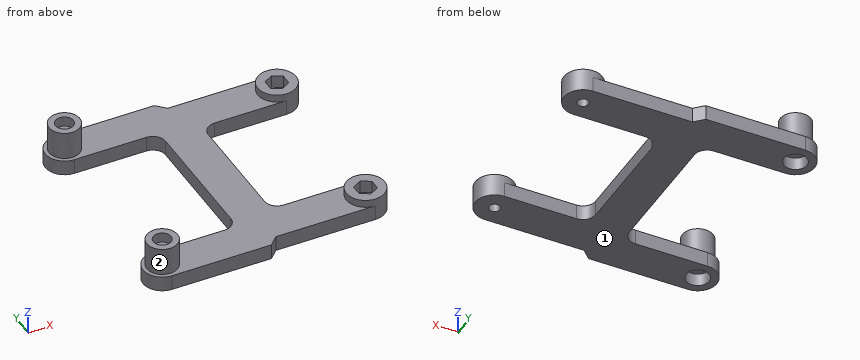
```python
from build123d import *

# Parameters (mm, degrees)
SKETCH1_R           = 4.5
SKETCH1_R_2         = 2.15
BOSS_EXTRUDE1_DEPTH = 6
BOSS_EXTRUDE2_START = -1
SKETCH2_R           = 6
SKETCH2_R_2         = 3.5
BOSS_EXTRUDE2_DEPTH = 12
BOSS_EXTRUDE3_START = -5
SKETCH3_R           = 3.5
SKETCH3_R_2         = 1.65
BOSS_EXTRUDE3_DEPTH = 8
SKETCH4_R           = 7.5
SKETCH4_R_2         = 2.15
BOSS_EXTRUDE4_DEPTH = 3
CUT_EXTRUDE1_DEPTH  = 5


with BuildPart() as part:
    # Sketch1 → Boss-Extrude1 (new body)
    with BuildSketch(Plane.XY):
        with BuildLine():
            Line((0, 82.5), (39, 82.5))
            Line((39, 82.5), (42.5, 79))
            Line((42.5, 79), (81.5, 79))
            ThreePointArc((81.5, 79), (89, 71.5), (81.5, 64))
            Line((81.5, 64), (53.25, 64))
            ThreePointArc((53.25, 64), (49.714466094, 62.535533906), (48.25, 59))
            Line((48.25, 59), (48.25, 16))
            ThreePointArc((48.25, 16), (49.714466094, 12.464466094), (53.25, 11))
            Line((53.25, 11), (81.5, 11))
            ThreePointArc((81.5, 11), (89, 3.5), (81.5, -4))
            Line((81.5, -4), (42.5, -4))
            Line((42.5, -4), (39, -7.5))
            Line((39, -7.5), (0, -7.5))
            ThreePointArc((0, -7.5), (-7.5, 0), (0, 7.5))
            Line((0, 7.5), (28.25, 7.5))
            ThreePointArc((28.25, 7.5), (31.785533906, 8.964466094), (33.25, 12.5))
            Line((33.25, 12.5), (33.25, 62.5))
            ThreePointArc((33.25, 62.5), (31.785533906, 66.035533906), (28.25, 67.5))
            Line((28.25, 67.5), (0, 67.5))
            ThreePointArc((0, 67.5), (-7.5, 75), (0, 82.5))
        make_face()
        Circle(SKETCH1_R, mode=Mode.SUBTRACT)
        with Locations(Location((0, 75, 0), (0, 0, 180))):
            Circle(SKETCH1_R, mode=Mode.SUBTRACT)
        with Locations((81.5, 71.5)):
            Circle(SKETCH1_R_2, mode=Mode.SUBTRACT)
        with Locations((81.5, 3.5)):
            Circle(SKETCH1_R_2, mode=Mode.SUBTRACT)
    extrude(amount=BOSS_EXTRUDE1_DEPTH)

    # Sketch2 → Boss-Extrude2 (add)
    # profile 1 of 2: a face of its own
    with BuildSketch(Plane.XY.offset(6).offset(BOSS_EXTRUDE2_START)):
        with Locations(Location((0, 75, 0), (0, 0, 180))):
            Circle(SKETCH2_R)
        with Locations((0, 75)):
            Circle(SKETCH2_R_2, mode=Mode.SUBTRACT)
    # profile 2 of 2: a face of its own
    with BuildSketch(Plane.XY.offset(6).offset(BOSS_EXTRUDE2_START)):
        with Locations(Location((0, 0, 0), (0, 0, 180))):
            Circle(SKETCH2_R)
        Circle(SKETCH2_R_2, mode=Mode.SUBTRACT)
    extrude(amount=BOSS_EXTRUDE2_DEPTH)

    # Sketch3 → Boss-Extrude3 (add)
    # profile 1 of 2: a face of its own
    with BuildSketch(Plane(origin=(0, 0, 0), x_dir=(-1, 0, 0), z_dir=(0, 0, -1)).offset(BOSS_EXTRUDE3_START)):
        with Locations(Location((0, 75, 0), (0, 0, 180))):
            Circle(SKETCH3_R)
        with Locations((0, 75)):
            Circle(SKETCH3_R_2, mode=Mode.SUBTRACT)
    # profile 2 of 2: a face of its own
    with BuildSketch(Plane(origin=(0, 0, 0), x_dir=(-1, 0, 0), z_dir=(0, 0, -1)).offset(BOSS_EXTRUDE3_START)):
        with Locations(Location((0, 0, 0), (0, 0, 180))):
            Circle(SKETCH3_R)
        Circle(SKETCH3_R_2, mode=Mode.SUBTRACT)
    extrude(amount=-BOSS_EXTRUDE3_DEPTH)

    # Sketch4 → Boss-Extrude4 (add)
    # profile 1 of 2: a face of its own
    with BuildSketch(Plane.XY.offset(6)):
        with Locations(Location((81.5, 3.5, 0), (0, 0, 90))):
            Circle(SKETCH4_R)
        with Locations((81.5, 3.5)):
            Circle(SKETCH4_R_2, mode=Mode.SUBTRACT)
    # profile 2 of 2: a face of its own
    with BuildSketch(Plane.XY.offset(6)):
        with Locations(Location((81.5, 71.5, 0), (0, 0, 90))):
            Circle(SKETCH4_R)
        with Locations((81.5, 71.5)):
            Circle(SKETCH4_R_2, mode=Mode.SUBTRACT)
    extrude(amount=BOSS_EXTRUDE4_DEPTH)

    # Sketch5 → Cut-Extrude1 (cut)
    with BuildSketch(Plane.XY.offset(9)):
        Polygon((77.9, 5.578460969), (81.5, 7.656921938), (85.1, 5.578460969), (85.1, 1.421539031), (81.5, -0.656921938), (77.9, 1.421539031), align=None)
        Polygon((77.9, 73.578460969), (81.5, 75.656921938), (85.1, 73.578460969), (85.1, 69.421539031), (81.5, 67.343078062), (77.9, 69.421539031), align=None)
    extrude(amount=-CUT_EXTRUDE1_DEPTH, mode=Mode.SUBTRACT)


solid = part.part
```
Geometry check sheet. Reference: the model listing, model coordinates, mm. Face numbers are marked on the shaded views. Coordinates: 2 decimals unless noted, no trailing zeros. Order: outer loops, then holes, each group sorted by start corner. A loop starts at its lowest first (then second) coordinate and runs counter-clockwise, first axis right, second up.
Q1. Draft check along Y on the marked faces 1 and 2. Enter one of: released by +Y, released by -Y, zero draft, split by the parting line, or undercut.
Reply:
face 1: zero draft
face 2: undercut
Q2. Sectioned sample at C-C on y = 25. Record the cut outline in (x, z), and give its area (3 significant figures).
Reply:
outline: (33.25, 0) - (48.25, 0) - (48.25, 6) - (33.25, 6) - close
area: 90.0 mm2
Q3. Sectioned sample at A-A on x = 60. Record the cut outline in (y, z), and give its area (3 significant figures).
Reply:
outline: (-4, 0) - (11, 0) - (11, 6) - (-4, 6) - close; (64, 0) - (79, 0) - (79, 6) - (64, 6) - close
area: 180 mm2
Q4. Depth check by flat-ended pin: pin 1 Ø8 at (x, z) = (76.5, 5.5) entering from +Y; pin 2 Ø1.8 at (x, z) = (55.5, 2.5) entering from -Y; pin 3 Ø1.5 at (x, y) = (49.5, 32) entering from -Z; pin 4 Ø2 at (x, y) = (0, -1) entering from +Z. Enter the tip coordinate at first touch or a pass-through.
Reply:
pin 1: stops at y = 79
pin 2: stops at y = -4
pin 3: passes through
pin 4: stops at z = 13
Q5. Thickness scan on probe 1 along Y at (x, z) = (0, 1.2); probe 2 along Y at (x, z) = (81.5, 2.75); probe 3 along Y at (x, z) = (74.5, 3.5). Record the ranges inside material, lowest first.
Reply:
probe 1: y = -7.5 to -4.5, 4.5 to 7.5, 67.5 to 70.5, 79.5 to 82.5
probe 2: y = -4 to 1.35, 5.65 to 11, 64 to 69.35, 73.65 to 79
probe 3: y = -4 to 11, 64 to 79
Q6. Sectioned sample at B-B on z = 1.5. Record the cut outline in (x, y).
Reply:
outline: (0, -7.5) - (39, -7.5) - (42.5, -4) - (81.5, -4) arc R7.5 ccw to (81.5, 11) - (53.25, 11) arc R5 cw to (48.25, 16) - (48.25, 59) arc R5 cw to (53.25, 64) - (81.5, 64) arc R7.5 ccw to (81.5, 79) - (42.5, 79) - (39, 82.5) - (0, 82.5) arc R7.5 ccw to (0, 67.5) - (28.25, 67.5) arc R5 cw to (33.25, 62.5) - (33.25, 12.5) arc R5 cw to (28.25, 7.5) - (0, 7.5) arc R7.5 ccw to start; hole circle Ø9 at (0, 0); hole circle Ø9 at (0, 75); hole circle Ø4.3 at (81.5, 3.5); hole circle Ø4.3 at (81.5, 71.5)
